The listing builds one solid part. Answer for the finished solid, in the listing's coordinates (mm). Face numbers are marked on the shaded views. A direction names the side the tool comes from. Coordinates: 2 decimals unless noted, no trailing zeros. Loops run counter-clockwise (first coordinate to the right, second up) from the corner with the lowest first, then second, coordinate; pieces in that order, holes last. Notation, with made-up numbers: M 57.5,-20.5 L 87.5,-20.5 A10 ccw 87.5,-13.5 Z; hole C -36.5,-31 d9. An arc over 180 degrees is marked long. Return JSON: item names as keys, results as strings. Group by question number.
1. Straight lines are drawn through the part: L1, parallel to X at y = 1.5, z = 2.5; L2, parallel to X at y = 0.75, z = -1.5; L3, parallel to Y at x = -0.5, z = 0.75. For each, find the intervals that lie inside material, in ascending order. Write a range as from..to.
2. The mould has two halves that part along X. Classify the marked faces 3, 4 and 5: pulls with the +X half, pulls with the -X half, needs draft (parallel to the pull), parting line crosses it, or undercut.
3. Given P1, Ø2, axis at y = 8.5, z = -2, coming from the -X side; P2, Ø2, axis at y = 7, z = -1, coming from the +X side; P3, Ø1.5, axis at x = 0, y = 4.5, coming from the -Z side, each flat-ended and moving along its own axis, determine where each tip first touches the part or whether it passes through.
4. Section A-A (z = 0) is taken. Write down the section's boundary in (x, y) (3 decimals).
5. Which of the six approach directions +Z, -Z, +X, -X, +Y, -Y give full straight-line access (tool end or side, diameter ignored) to the marked faces 1 and 2?
6. Section B-B (x = 0) is taken. Write down the section's boundary in (y, z) (3 decimals).
7. Section D-D (y = 6) is taken. Write down the section's boundary in (x, z), then the cut area to 3 significant figures.
8. Section C-C (y = 1.25) is taken. Write down the section's boundary in (x, z), then the cut area to 3 significant figures.
```python
from build123d import *

# Parameters (mm, degrees)
SKETCH001_W  = 11
SKETCH001_H  = 1.6
POCKET_DEPTH = 1.6


with BuildPart() as part:
    # Sketch → Revolution (revolve)
    with BuildSketch(Plane.YZ):
        Polygon((0, 0), (0, 5.5), (0.5, 5.5), (3, 3), (9.64493, 3), (10, 2.385), (10, 0), align=None)
    revolve(axis=Axis((0, 0, 0), (0, 1, 0)))

    # Sketch001 → Pocket (cut)
    with BuildSketch(Plane(origin=(0, 0, 0), x_dir=(0, 0, -1), z_dir=(0, -1, 0))):
        Rectangle(SKETCH001_W, SKETCH001_H)
    extrude(amount=-POCKET_DEPTH, mode=Mode.SUBTRACT)


solid = part.part
```
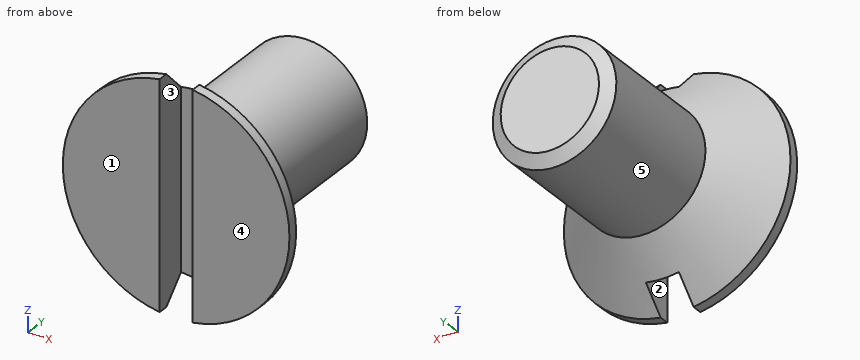
Worked out:
{
 "1": {"L1": "-3.74..-0.8, 0.8..3.74", "L2": "-5.03..-0.8, 0.8..5.03", "L3": "1.6..10"},
 "2": {"face 3": "undercut", "face 4": "needs draft", "face 5": "parting line crosses it"},
 "3": {"P1": "x = -2.83", "P2": "x = 3", "P3": "z = -3"},
 "4": {"outline": "M -5.5,0 L -0.8,0 L -0.8,1.6 L 0.8,1.6 L 0.8,0 L 5.5,0 L 5.5,0.5 L 3,3 L 3,9.645 L 2.385,10 L -2.385,10 L -3,9.645 L -3,3 L -5.5,0.5 Z"},
 "5": {"face 1": "+Z, -Z, +X, -X, -Y", "face 2": "+Z, -Z, -Y"},
 "6": {"outline": "M 1.6,-4.4 L 3,-3 L 9.645,-3 L 10,-2.385 L 10,2.385 L 9.645,3 L 3,3 L 1.6,4.4 Z"},
 "7": {"outline": "C 0,0 d6", "area": "28.3 mm^2"},
 "8": {"outline": "M -0.8,-4.68 L -0.8,4.68 A4.75 ccw Z; M 0.8,-4.68 A4.75 ccw 0.8,4.68 Z", "area": "55.8 mm^2"}
}
